Can you work these out from the drawing? Everything is in mm from the part's minimum corner. A direction names the side the tool comes from. Give positions to 0.01 mm unless a question says otherwise; leave off trailing zeros. Write each loop counter-clockwise with the first axis right and the second up, starting at its lowest first coordinate (ties: lowest second). Pieces come first, ordered by that corner, then holes. Notation, with made-up numbers: (9, 81.5) - (23, 81.5) arc R34 ccw to (23, 111.5) - close; hole circle Ø3 at (20, 23.5). An arc over 180 degrees is marked (long way). Use a Markdown table: item, result.
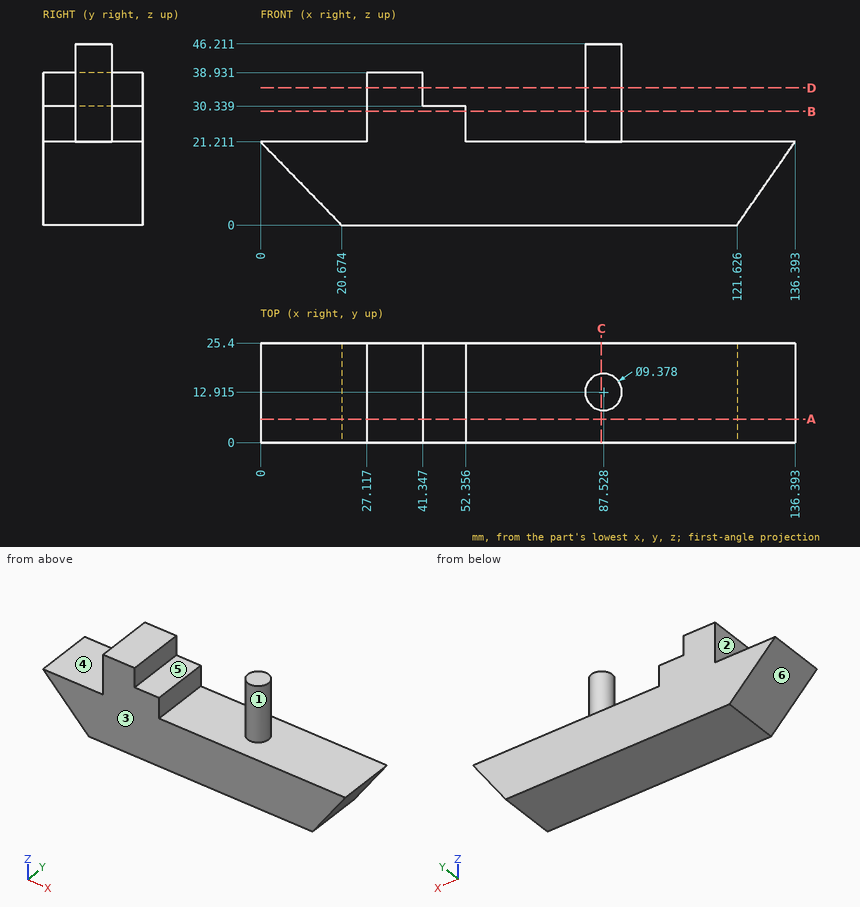
Item 1: Thinking about a two-plate mould opening in X: for the marked faces 1, 2 and 3, which applies, +X half, -X half, draft (parallel to the pull), parting line (faces both ways), or undercut?
Values:
| item | result |
|---|---|
| face 1 | undercut |
| face 2 | -X half |
| face 3 | draft |
Item 2: I need wall thicknesses on line 1 along X through (y, z) = (22.25, 31.5); line 2 along Z through (x, y) = (79, 9.75); line 3 along Z through (x, y) = (51, 20.25). Which ranges of each line are inside material? Lowest first, please. Write a range as [from, to].
Values:
| item | result |
|---|---|
| line 1 | x = [27.12, 41.35] |
| line 2 | z = [0, 21.21] |
| line 3 | z = [0, 30.34] |
Item 3: If we section it at D-D, the plane z = 35: Write out the boundary of the cut face in (x, y) (1 decimal).
Values:
| item | result |
|---|---|
| outline | (27.1, 0) - (41.3, 0) - (41.3, 25.4) - (27.1, 25.4) - close; circle Ø9.4 at (87.5, 12.9) |
Item 4: For the marked faces 4, 5 and 6, which set-ups out of +Z, -Z, +X, -X, +Y, -Y let a thin tool reach every point of the face, with its end or its side?
Values:
| item | result |
|---|---|
| face 4 | +Z, -X, +Y, -Y |
| face 5 | +Z, +Y, -Y |
| face 6 | -Z, -X, +Y, -Y |
Item 5: Will these pins go through, and if not, where does the flat tip stop? pin 1 Ø1 at (y, z) = (22, 31) entering from +X; pin 2 Ø6 at (x, y) = (109, 19.5) entering from +Z; pin 3 Ø6 at (x, z) = (25.5, 39) entering from -Y; pin 4 Ø4.5 at (x, y) = (33, 12.5) entering from +Z.
Values:
| item | result |
|---|---|
| pin 1 | stops at x = 41.35 |
| pin 2 | stops at z = 21.21 |
| pin 3 | stops at y = 0 |
| pin 4 | stops at z = 38.93 |
Item 6: If we section it at B-B, the plane z = 29: Write out the boundary of the cut face in (x, y) (1 decimal), plus the area to 3 significant figures.
Values:
| item | result |
|---|---|
| outline | (27.1, 0) - (52.4, 0) - (52.4, 25.4) - (27.1, 25.4) - close; circle Ø9.4 at (87.5, 12.9) |
| area | 710 mm2 |
Item 7: If we section it at C-C, the plane x = 87: Write out the boundary of the cut face in (y, z) (1 decimal), plus the area to 3 significant figures.
Values:
| item | result |
|---|---|
| outline | (0, 0) - (25.4, 0) - (25.4, 21.2) - (17.6, 21.2) - (17.6, 46.2) - (8.3, 46.2) - (8.3, 21.2) - (0, 21.2) - close |
| area | 772 mm2 |
Item 8: If we section it at A-A, the plane y = 6: Write out the boundary of the cut face in (x, z) (1 decimal), plus the area to 3 significant figures.
Values:
| item | result |
|---|---|
| outline | (0, 21.2) - (20.7, 0) - (121.6, 0) - (136.4, 21.2) - (52.4, 21.2) - (52.4, 30.3) - (41.3, 30.3) - (41.3, 38.9) - (27.1, 38.9) - (27.1, 21.2) - close |
| area | 2,870 mm2 |
